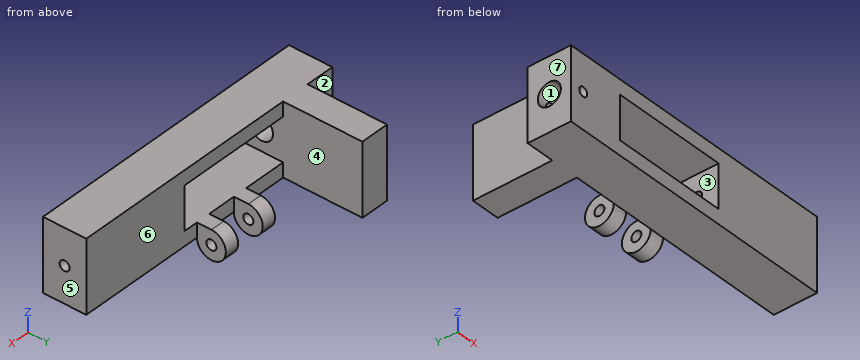
```python
from build123d import *

# Parameters (mm, degrees)
SKETCH2_W                            = 100
SKETCH2_H                            = 25
SKETCH2_W_2                          = 40
SKETCH2_H_2                          = 15
BOSS_EXTRUDE1_DEPTH                  = 15
CUT_EXTRUDE1_REACH                   = 103.888
SKETCH3_R                            = 1.75
CUT_EXTRUDE2_REACH                   = 103.888
SKETCH4_R                            = 4
F_3_2_3_2_DIAMETER_HOLE1_D           = 3.2
F_3_2_3_2_DIAMETER_HOLE1_CSINK_D     = 3.25
F_3_2_3_2_DIAMETER_HOLE1_CSINK_ANGLE = 90
SKETCH8_W                            = 10
SKETCH8_H                            = 25
BOSS_EXTRUDE2_DEPTH                  = 27.5
SKETCH9_R                            = 1.75
BOSS_EXTRUDE3_DEPTH                  = 40
CUT_EXTRUDE3_REACH                   = 70.283
SKETCH10_W                           = 15
SKETCH10_H                           = 10
SKETCH10_W_2                         = 10
SKETCH10_W_3                         = 5


with BuildPart() as part:
    # Sketch2 → Boss-Extrude1 (new body)
    with BuildSketch(Plane(origin=(0, 0, 0), x_dir=(1, 0, 0), z_dir=(0, 1, 0))):
        with Locations((10, 0)):
            Rectangle(SKETCH2_W, SKETCH2_H)
        Rectangle(SKETCH2_W_2, SKETCH2_H_2, mode=Mode.SUBTRACT)
    extrude(amount=BOSS_EXTRUDE1_DEPTH)

    # Sketch3 → Cut-Extrude1 (cut, up to next)
    with BuildSketch(Plane(origin=(60, 0, 0), x_dir=(0, 0, -1), z_dir=(1, 0, 0)), mode=Mode.PRIVATE) as cut_extrude1_sk1:
        with Locations((0, 7.5)):
            Circle(SKETCH3_R)
    cut_extrude1_tool1 = extrude(cut_extrude1_sk1.sketch, amount=-CUT_EXTRUDE1_REACH, mode=Mode.PRIVATE) & part.part
    add(cut_extrude1_tool1.solids().sort_by_distance((60, 7.5, 0))[0], mode=Mode.SUBTRACT)

    # Sketch4 → Cut-Extrude2 (cut, up to next)
    with BuildSketch(Plane.ZY.offset(40), mode=Mode.PRIVATE) as cut_extrude2_sk1:
        with Locations((0, 7.5)):
            Circle(SKETCH4_R)
    cut_extrude2_tool1 = extrude(cut_extrude2_sk1.sketch, amount=-CUT_EXTRUDE2_REACH, mode=Mode.PRIVATE) & part.part
    add(cut_extrude2_tool1.solids().sort_by_distance((-40, 7.5, 0))[0], mode=Mode.SUBTRACT)

    # Ø3.2 (3.2) Diameter Hole1 (through all)
    with Locations(Plane(origin=(0, 15, 0), x_dir=(1, 0, 0), z_dir=(0, 1, 0))):
        with Locations((-35, 0)):
            CounterSinkHole(F_3_2_3_2_DIAMETER_HOLE1_D / 2, F_3_2_3_2_DIAMETER_HOLE1_CSINK_D / 2, counter_sink_angle=F_3_2_3_2_DIAMETER_HOLE1_CSINK_ANGLE)

    # Sketch8 → Boss-Extrude2 (add)
    with BuildSketch(Plane(origin=(0, 15, 0), x_dir=(1, 0, 0), z_dir=(0, 1, 0))):
        with Locations((-25, 0)):
            Rectangle(SKETCH8_W, SKETCH8_H)
    extrude(amount=BOSS_EXTRUDE2_DEPTH)

    # Sketch9 → Boss-Extrude3 (add)
    with BuildSketch(Plane(origin=(-20, 0, 0), x_dir=(0, 0, -1), z_dir=(1, 0, 0))):
        with BuildLine():
            Line((7.5, 20), (7.5, 15))
            Line((7.5, 15), (12.5, 15))
            ThreePointArc((12.5, 15), (16.035533906, 23.535533906), (7.5, 20))
        make_face()
        with Locations(Location((12.5, 20, 0), (0, 0, 90))):
            Circle(SKETCH9_R, mode=Mode.SUBTRACT)
    extrude(amount=BOSS_EXTRUDE3_DEPTH)

    # Sketch10 → Cut-Extrude3 (cut, up to next)
    with BuildSketch(Plane(origin=(0, 15, 0), x_dir=(1, 0, 0), z_dir=(0, 1, 0)), mode=Mode.PRIVATE) as cut_extrude3_sk1:
        with Locations((-12.5, 12.5)):
            Rectangle(SKETCH10_W, SKETCH10_H)
    cut_extrude3_tool1 = extrude(cut_extrude3_sk1.sketch, amount=CUT_EXTRUDE3_REACH, mode=Mode.PRIVATE) & part.part
    # Sketch10 → Cut-Extrude3 (cut, up to next)
    with BuildSketch(Plane(origin=(0, 15, 0), x_dir=(1, 0, 0), z_dir=(0, 1, 0)), mode=Mode.PRIVATE) as cut_extrude3_sk2:
        with Locations((5, 12.5)):
            Rectangle(SKETCH10_W_2, SKETCH10_H)
    cut_extrude3_tool2 = extrude(cut_extrude3_sk2.sketch, amount=CUT_EXTRUDE3_REACH, mode=Mode.PRIVATE) & part.part
    # Sketch10 → Cut-Extrude3 (cut, up to next)
    with BuildSketch(Plane(origin=(0, 15, 0), x_dir=(1, 0, 0), z_dir=(0, 1, 0)), mode=Mode.PRIVATE) as cut_extrude3_sk3:
        with Locations((17.5, 12.5)):
            Rectangle(SKETCH10_W_3, SKETCH10_H)
    cut_extrude3_tool3 = extrude(cut_extrude3_sk3.sketch, amount=CUT_EXTRUDE3_REACH, mode=Mode.PRIVATE) & part.part
    add(cut_extrude3_tool1.solids().sort_by_distance((-12.5, 15, -12.5))[0], mode=Mode.SUBTRACT)
    add(cut_extrude3_tool2.solids().sort_by_distance((5, 15, -12.5))[0], mode=Mode.SUBTRACT)
    add(cut_extrude3_tool3.solids().sort_by_distance((17.5, 15, -12.5))[0], mode=Mode.SUBTRACT)


solid = part.part
```
The model under review builds one solid part; all positions refer to its coordinate system, in mm. Face numbers are marked on the shaded views. A direction names the side the tool comes from. Round coordinates to 2 decimals unless told otherwise and drop trailing zeros. Order: outer loops, then holes, each group sorted by start corner. A loop starts at its lowest first (then second) coordinate and runs counter-clockwise, first axis right, second up.
Item 1: For pin 1 (3 mm diameter, centred on y = 37, z = -11, fed in from +X); pin 2 (5.5 mm diameter, centred on x = 4.5, z = -10, fed in from +Y); pin 3 (12 mm diameter, centred on x = 7, y = 7.5, fed in from -Z), all flat-tipped, find the tip position at first contact; note any pin that passes through.
Working result:
pin 1: stops at x = -20
pin 2: stops at y = 15
pin 3: stops at z = -12.5
Item 2: Draft analysis for pull direction X (two halves, no side actions). For the marked faces 4, 5, 6 and 7, state which applies: released by +X, released by -X, zero draft, split by the parting line, or undercut.
Working result:
face 4: undercut
face 5: released by +X
face 6: zero draft
face 7: released by -X
Item 3: Machinability: for the marked faces 1, 2 and 3, which of the approach directions +Z, -Z, +X, -X, +Y, -Y give a long, thin tool a straight path to every point of the face, cutting with its end or side? Answer none if there is none.
Working result:
face 1: -X
face 2: +Z, -Z, -X, +Y
face 3: +Y, -Y
Item 4: Add section A-A, the plane x = -2. State the section outline as (y, z) points.
Working result:
outline: (0, -12.5) - (15, -12.5) arc R5 ccw (long way) to (20, -7.5) - (0, -7.5) - close; (0, 7.5) - (15, 7.5) - (15, 12.5) - (0, 12.5) - close; hole circle Ø3.5 at (20, -12.5)
Item 5: Add section B-B, the plane z = -6.5. State the section outline as (x, y) points.
Working result:
outline: (-40, 0) - (-20, 0) - (-20, 42.5) - (-30, 42.5) - (-30, 15) - (-40, 15) - close; (20, 0) - (60, 0) - (60, 15) - (20, 15) - close
Item 6: Add section D-D, the plane z = 0. State the section outline as (x, y) points (3 decimals).
Working result:
outline: (-40, 0) - (-36.6, 0) - (-36.6, 3.5) - (-40, 3.5) - close; (-40, 11.5) - (-36.6, 11.5) - (-36.6, 14.975) - (-36.625, 15) - (-40, 15) - close; (-33.4, 0) - (-20, 0) - (-20, 3.5) - (-33.4, 3.5) - close; (-33.4, 11.5) - (-20, 11.5) - (-20, 42.5) - (-30, 42.5) - (-30, 15) - (-33.375, 15) - (-33.4, 14.975) - close; (20, 0) - (60, 0) - (60, 5.75) - (20, 5.75) - close; (20, 9.25) - (60, 9.25) - (60, 15) - (20, 15) - close
Item 7: To check wall thickness, follow probe 1 along X at (y, z) = (17, -10); probe 2 along Z at (x, y) = (-35, 13.8); probe 3 along Y at (x, z) = (30.5, 0). State the ranges of each line that lie inside material, in increasing order.
Working result:
probe 1: x = -30 to -20, -5 to 0, 10 to 15
probe 2: z = -12.5 to -1.6, 1.6 to 12.5
probe 3: y = 0 to 5.75, 9.25 to 15
Item 8: Add section C-C, the plane x = -35. State the section outline as (y, z) points (3 decimals).
Working result:
outline: (0, -12.5) - (15, -12.5) - (15, -1.625) - (14.975, -1.6) - (11.166, -1.6) arc R4 cw to (3.834, -1.6) - (0, -1.6) - close; (0, 1.6) - (3.834, 1.6) arc R4 cw to (11.166, 1.6) - (14.975, 1.6) - (15, 1.625) - (15, 12.5) - (0, 12.5) - close
